```python
from build123d import *

# Parameters (mm, degrees)
SKETCH2_R           = 1.45
SKETCH2_R_2         = 1.25
BOSS_EXTRUDE1_DEPTH = 1.35
CUT_EXTRUDE1_REACH  = 74.065
SKETCH5_RX          = 10.25
SKETCH5_RY          = 6.825
SKETCH5_W           = 3.5
SKETCH5_H           = 16.5


with BuildPart() as part:
    # Sketch2 → Boss-Extrude1 (new body)
    with BuildSketch(Plane(origin=(0, 0, 0), x_dir=(1, 0, 0), z_dir=(0, 1, 0))):
        with BuildLine():
            Line((-29.305, -34.965), (29.305, -34.965))
            ThreePointArc((29.305, -34.965), (30.719213562, -34.379213562), (31.305, -32.965))
            Line((31.305, -32.965), (31.305, -20.75))
            ThreePointArc((31.305, -20.75), (32.769466094, -17.214466094), (36.305, -15.75))
            Line((36.305, -15.75), (61, -15.75))
            ThreePointArc((61, -15.75), (62.414213562, -15.164213562), (63, -13.75))
            Line((63, -13.75), (63, 13.75))
            ThreePointArc((63, 13.75), (62.414213562, 15.164213562), (61, 15.75))
            Line((61, 15.75), (36.305, 15.75))
            ThreePointArc((36.305, 15.75), (32.769466094, 17.214466094), (31.305, 20.75))
            Line((31.305, 20.75), (31.305, 32.965))
            ThreePointArc((31.305, 32.965), (30.719213562, 34.379213562), (29.305, 34.965))
            Line((29.305, 34.965), (-29.305, 34.965))
            ThreePointArc((-29.305, 34.965), (-30.719213562, 34.379213562), (-31.305, 32.965))
            Line((-31.305, 32.965), (-31.305, 20.75))
            ThreePointArc((-31.305, 20.75), (-32.769466094, 17.214466094), (-36.305, 15.75))
            Line((-36.305, 15.75), (-61, 15.75))
            ThreePointArc((-61, 15.75), (-62.414213562, 15.164213562), (-63, 13.75))
            Line((-63, 13.75), (-63, -13.75))
            ThreePointArc((-63, -13.75), (-62.414213562, -15.164213562), (-61, -15.75))
            Line((-61, -15.75), (-36.305, -15.75))
            ThreePointArc((-36.305, -15.75), (-32.769466094, -17.214466094), (-31.305, -20.75))
            Line((-31.305, -20.75), (-31.305, -32.965))
            ThreePointArc((-31.305, -32.965), (-30.719213562, -34.379213562), (-29.305, -34.965))
        make_face()
        with Locations(Location((21, -10.75, 0), (0, 0, 270))):
            Circle(SKETCH2_R, mode=Mode.SUBTRACT)
        with Locations(Location((21, 10.75, 0), (0, 0, 270))):
            Circle(SKETCH2_R, mode=Mode.SUBTRACT)
        with Locations(Location((-21, 10.75, 0), (0, 0, 270))):
            Circle(SKETCH2_R, mode=Mode.SUBTRACT)
        with Locations(Location((-24.5, 29.84, 0), (0, 0, 270))):
            Circle(SKETCH2_R_2, mode=Mode.SUBTRACT)
        with Locations(Location((-21, -10.75, 0), (0, 0, 270))):
            Circle(SKETCH2_R, mode=Mode.SUBTRACT)
        with Locations(Location((-24.5, -28.16, 0), (0, 0, 270))):
            Circle(SKETCH2_R_2, mode=Mode.SUBTRACT)
        with Locations(Location((-57, -11.65, 0), (0, 0, 270))):
            Circle(SKETCH2_R_2, mode=Mode.SUBTRACT)
        with Locations(Location((24.5, -28.16, 0), (0, 0, 270))):
            Circle(SKETCH2_R_2, mode=Mode.SUBTRACT)
        with Locations(Location((-57, 11.65, 0), (0, 0, 270))):
            Circle(SKETCH2_R_2, mode=Mode.SUBTRACT)
        with Locations(Location((24.5, 29.84, 0), (0, 0, 270))):
            Circle(SKETCH2_R_2, mode=Mode.SUBTRACT)
        with Locations(Location((57, 11.65, 0), (0, 0, 270))):
            Circle(SKETCH2_R_2, mode=Mode.SUBTRACT)
        with Locations(Location((-37, 8.15, 0), (0, 0, 270))):
            Circle(SKETCH2_R_2, mode=Mode.SUBTRACT)
        with Locations(Location((-37, -8.15, 0), (0, 0, 270))):
            Circle(SKETCH2_R_2, mode=Mode.SUBTRACT)
        with Locations(Location((37, -8.15, 0), (0, 0, 270))):
            Circle(SKETCH2_R_2, mode=Mode.SUBTRACT)
        with Locations(Location((37, 8.15, 0), (0, 0, 270))):
            Circle(SKETCH2_R_2, mode=Mode.SUBTRACT)
        with Locations(Location((57, -11.65, 0), (0, 0, 270))):
            Circle(SKETCH2_R_2, mode=Mode.SUBTRACT)
    extrude(amount=-BOSS_EXTRUDE1_DEPTH)

    # Sketch5 → Cut-Extrude1 (cut, up to next)
    with BuildSketch(Plane(origin=(0, 0, 0), x_dir=(1, 0, 0), z_dir=(0, 1, 0)), mode=Mode.PRIVATE) as cut_extrude1_sk1:
        with Locations(Location((47.75, 0), (0, 0, 180))):
            Ellipse(SKETCH5_RX, SKETCH5_RY)
    cut_extrude1_tool1 = extrude(cut_extrude1_sk1.sketch, amount=-CUT_EXTRUDE1_REACH, mode=Mode.PRIVATE) & part.part
    # Sketch5 → Cut-Extrude1 (cut, up to next)
    with BuildSketch(Plane(origin=(0, 0, 0), x_dir=(1, 0, 0), z_dir=(0, 1, 0)), mode=Mode.PRIVATE) as cut_extrude1_sk2:
        with Locations(Location((-47.75, 0), (0, 0, 0))):
            Ellipse(SKETCH5_RX, SKETCH5_RY)
    cut_extrude1_tool2 = extrude(cut_extrude1_sk2.sketch, amount=-CUT_EXTRUDE1_REACH, mode=Mode.PRIVATE) & part.part
    # Sketch5 → Cut-Extrude1 (cut, up to next)
    with BuildSketch(Plane(origin=(0, 0, 0), x_dir=(1, 0, 0), z_dir=(0, 1, 0)), mode=Mode.PRIVATE) as cut_extrude1_sk3:
        with Locations((11.65, 0)):
            Rectangle(SKETCH5_W, SKETCH5_H)
    cut_extrude1_tool3 = extrude(cut_extrude1_sk3.sketch, amount=-CUT_EXTRUDE1_REACH, mode=Mode.PRIVATE) & part.part
    # Sketch5 → Cut-Extrude1 (cut, up to next)
    with BuildSketch(Plane(origin=(0, 0, 0), x_dir=(1, 0, 0), z_dir=(0, 1, 0)), mode=Mode.PRIVATE) as cut_extrude1_sk4:
        with Locations((-11.65, 0)):
            Rectangle(SKETCH5_W, SKETCH5_H)
    cut_extrude1_tool4 = extrude(cut_extrude1_sk4.sketch, amount=-CUT_EXTRUDE1_REACH, mode=Mode.PRIVATE) & part.part
    add(cut_extrude1_tool1.solids().sort_by_distance((47.75, 0, 0))[0], mode=Mode.SUBTRACT)
    add(cut_extrude1_tool2.solids().sort_by_distance((-47.75, 0, 0))[0], mode=Mode.SUBTRACT)
    add(cut_extrude1_tool3.solids().sort_by_distance((11.65, 0, 0))[0], mode=Mode.SUBTRACT)
    add(cut_extrude1_tool4.solids().sort_by_distance((-11.65, 0, 0))[0], mode=Mode.SUBTRACT)


solid = part.part
```
The listing builds one solid part. Answer for the finished solid, in the listing's coordinates (mm). Round coordinates to 2 decimals unless told otherwise and drop trailing zeros. Loops run counter-clockwise (first coordinate to the right, second up) from the corner with the lowest first, then second, coordinate; pieces in that order, holes last. Notation, with made-up numbers: (-5.5, 43.25) - (6.5, 43.25) arc R24 ccw to (6.5, 60.25) - close; hole circle Ø2 at (10, 19). An arc over 180 degrees is marked (long way). Return JSON: item names as keys, results as strings. Group by question number.
1. The part is cut by section C-C on y = -0.85. State how many separate pieces and enclosed holes the cut face has, then the cut area to 3 significant figures.
2. The part is cut by section B-B on z = 28.16. Determine the outline of the cut face in (x, y) (3 decimals), then the cut area to 3 significant figures.
3. The mould has two halves that part along X. Classify faces 1 (the cylindrical face through (33, -1, -17)), 2 (the cylindrical face through (-33, -1, -17)), 3 (the cylindrical face through (58.24, -0.67, -11.81)): pulls with the +X half, pulls with the -X half, needs draft (parallel to the pull), parting line crosses it, or undercut.
4. Consider probe 1 along X at (y, z) = (-0.8, -29.84) (3 decimals); probe 2 along X at (y, z) = (-0.9, -8.15); probe 3 along Z at (x, y) = (-12, -0.6) (3 decimals). Determine where each line is inside the solid, lowest interval first.
5. The part is cut by section A-A on x = -21. Determine the outline of the cut face in (y, z) (3 decimals).
Resolved:
{
 "1": {"separate pieces": "1", "enclosed holes": "20", "area": "5,750 mm²"},
 "2": {"outline": "(-31.305, -1.35) - (-25.75, -1.35) - (-25.75, 0) - (-31.305, 0) - close; (-23.25, -1.35) - (23.25, -1.35) - (23.25, 0) - (-23.25, 0) - close; (25.75, -1.35) - (31.305, -1.35) - (31.305, 0) - (25.75, 0) - close", "area": "77.8 mm²"},
 "3": {"face 1": "pulls with the +X half", "face 2": "pulls with the -X half", "face 3": "undercut"},
 "4": {"probe 1": "x = -31.305 to -25.75, -23.25 to 23.25, 25.75 to 31.305", "probe 2": "x = -63 to -38.25, -35.75 to -13.4, -9.9 to 9.9, 13.4 to 35.75, 38.25 to 63", "probe 3": "z = -34.965 to -8.25, 8.25 to 34.965"},
 "5": {"outline": "(-1.35, -34.965) - (0, -34.965) - (0, -12.2) - (-1.35, -12.2) - close; (-1.35, -9.3) - (0, -9.3) - (0, 9.3) - (-1.35, 9.3) - close; (-1.35, 12.2) - (0, 12.2) - (0, 34.965) - (-1.35, 34.965) - close"}
}
